Could you check a few things on this drawing? It's one solid part, dimensions in mm from its lowest x, y, z. A direction names the side the tool comes from. Give positions to 0.01 mm unless a question says otherwise; leave off trailing zeros. Loops run counter-clockwise (first coordinate to the right, second up) from the corner with the lowest first, then second, coordinate; pieces in that order, holes last. Notation, with made-up numbers: M 22.25,-2 L 71.25,-2 A10 ccw 71.25,13 Z; hole C 61,86.5 d11. An arc over 180 degrees is marked long. Answer as a JSON object with one key per item and string values.
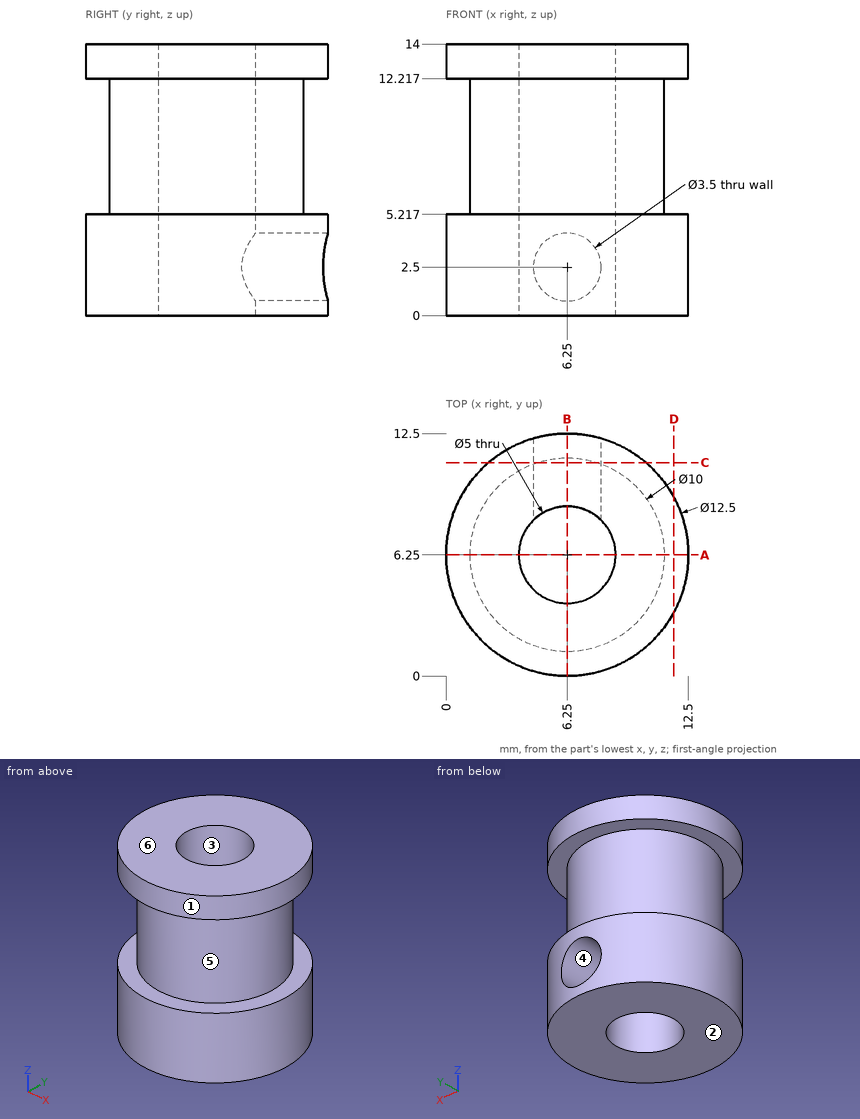
1) Suppose I cut it at A-A, the plane y = 6.25. Write out the boundary of the cut face in (x, z).
Answer list:
{"outline": "M 0,0 L 3.75,0 L 3.75,14 L 0,14 L 0,12.22 L 1.25,12.22 L 1.25,5.22 L 0,5.22 Z; M 8.75,0 L 12.5,0 L 12.5,5.22 L 11.25,5.22 L 11.25,12.22 L 12.5,12.22 L 12.5,14 L 8.75,14 Z"}
2) If we mould it in two halves opening along Y, with no side actions, what happens to the marked faces 1, 2 and 3? For each: +Y half, -Y half, draft (parallel to the pull), parting line (faces both ways), or undercut.
Answer list:
{"face 1": "parting line", "face 2": "draft", "face 3": "undercut"}
3) Suppose I cut it at D-D, the plane x = 11.75. Write out the boundary of the cut face in (y, z), and give its area (3 significant figures).
Answer list:
{"outline": "M 3.28,0 L 9.22,0 L 9.22,5.22 L 3.28,5.22 Z; M 3.28,12.22 L 9.22,12.22 L 9.22,14 L 3.28,14 Z", "area": "41.6 mm^2"}
4) Please list where these lines run through material, in increasing order: line 1 along Z through (x, y) = (6.25, 10.9); line 2 along Y through (x, z) = (6.25, 8.25); line 3 along X through (y, z) = (2.5, 2). Write a range as from..to.
Answer list:
{"line 1": "0..0.75, 4.25..14", "line 2": "1.25..3.75, 8.75..11.25", "line 3": "1.25..11.25"}
5) Will these pins go through, and if not, where does the flat tip stop? pin 1 Ø4 at (y, z) = (10, 4) entering from -X; pin 2 Ø1 at (y, z) = (9, 11) entering from +X (3 decimals); pin 3 Ø3 at (x, z) = (6.25, 2.5) entering from +Y.
Answer list:
{"pin 1": "x = 0.25", "pin 2": "x = 10.715", "pin 3": "y = 4.25"}
6) For the marked faces 4, 5 and 6, which set-ups out of +Z, -Z, +X, -X, +Y, -Y let a thin tool reach every point of the face, with its end or its side?
Answer list:
{"face 4": "+Y", "face 5": "none", "face 6": "+Z, +X, -X, +Y, -Y"}
7) Suppose I cut it at B-B, the plane x = 6.25. Write out the boundary of the cut face in (y, z).
Answer list:
{"outline": "M 0,0 L 3.75,0 L 3.75,14 L 0,14 L 0,12.22 L 1.25,12.22 L 1.25,5.22 L 0,5.22 Z; M 8.75,0 L 12.5,0 L 12.5,0.75 L 8.75,0.75 Z; M 8.75,4.25 L 12.5,4.25 L 12.5,5.22 L 11.25,5.22 L 11.25,12.22 L 12.5,12.22 L 12.5,14 L 8.75,14 Z"}
8) Suppose I cut it at C-C, the plane y = 11. Write out the boundary of the cut face in (x, z).
Answer list:
{"outline": "M 2.19,0 L 10.31,0 L 10.31,5.22 L 7.81,5.22 L 7.81,12.22 L 10.31,12.22 L 10.31,14 L 2.19,14 L 2.19,12.22 L 4.69,12.22 L 4.69,5.22 L 2.19,5.22 Z; hole C 6.25,2.5 d3.5"}
